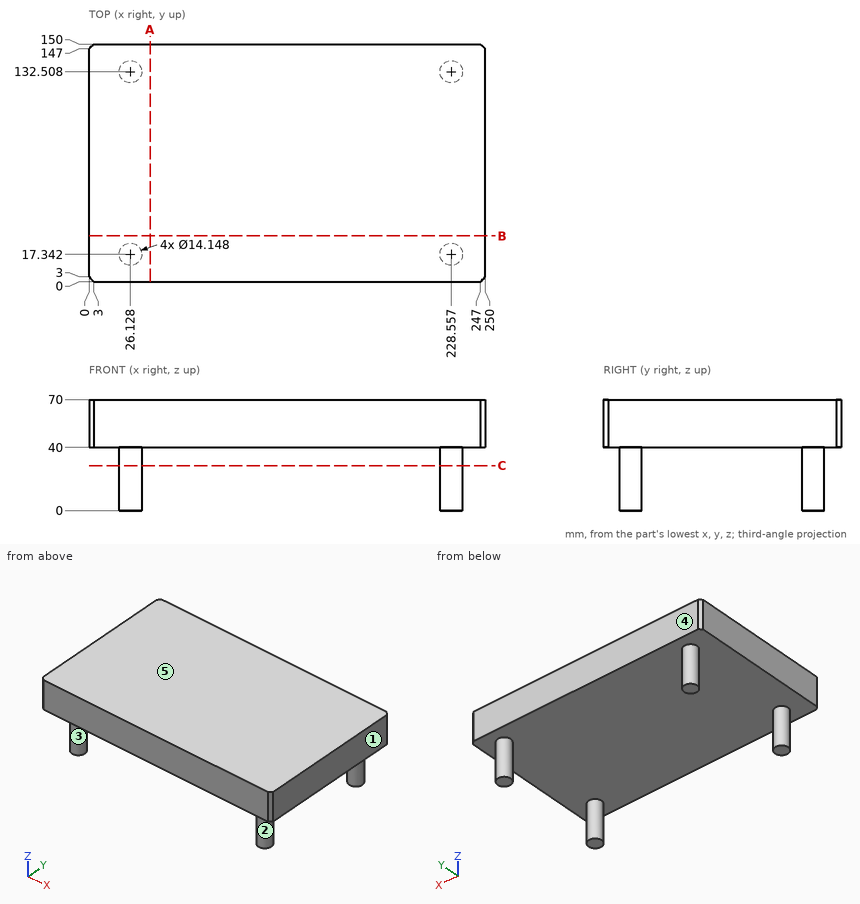
Can you work these out from the drawing? Everything is in mm from the part's minimum corner. A direction names the side the tool comes from. Coordinates: 2 decimals unless noted, no trailing zeros. Write each loop counter-clockwise with the first axis right and the second up, starting at its lowest first coordinate (ties: lowest second). Pieces come first, ordered by that corner, then holes. Notation, with made-up numbers: (40.25, 75) -> (60.25, 75) arc R11 ccw to (60.25, 89) -> close; hole circle Ø1 at (32.5, 79.25). An arc over 180 degrees is marked (long way). Return JSON: item names as keys, results as strings.
(1) Imagine slicing it at C-C, the plane z = 28.5. Please give me the cut outline in (x, y), then the cut area to 3 significant figures.
Numbers:
{"outline": "circle Ø14.15 at (26.13, 17.34); circle Ø14.15 at (26.13, 132.51); circle Ø14.15 at (228.56, 17.34); circle Ø14.15 at (228.56, 132.51)", "area": "629 mm2"}
(2) Imagine slicing it at A-A, the plane x = 38.5. Please give me the cut outline in (y, z), then the cut area to 3 significant figures.
Numbers:
{"outline": "(0, 40) -> (150, 40) -> (150, 70) -> (0, 70) -> close", "area": "4,500 mm2"}
(3) Which directions (+Z, -Z, +X, -X, +Y, -Y) give clear straight access to the entire face, cutting with the end or side of a thin tool? Please do the marked faces 1 and 2.
Numbers:
{"face 1": "+Z, -Z, +X, +Y, -Y", "face 2": "-Z"}
(4) We'd pull the mould along Y, two halves only. Please class the marked faces 3, 4 and 5: +Y half, -Y half, draft (parallel to the pull), parting line (faces both ways), or undercut.
Numbers:
{"face 3": "undercut", "face 4": "+Y half", "face 5": "draft"}
(5) I'm going to push a flat-ended pin straight in: pin 1 (2 mm diameter, centred on x = 109, y = 74, fed in from -Z). Where does the tip first touch, or does it pass through?
Numbers:
{"pin 1": "stops at z = 40"}
(6) Imagine slicing it at B-B, the plane y = 29. Please give me the cut outline in (x, z), then the cut area to 3 significant figures.
Numbers:
{"outline": "(0, 40) -> (250, 40) -> (250, 70) -> (0, 70) -> close", "area": "7,500 mm2"}
(7) I need wall thicknesses on L1, parallel to Z at x = 210, y = 50.5; L2, parallel to X at y = 16.5, z = 14.5; L3, parallel to Y at x = 25, z = 18 (1 decimal). Which ranges of each line are inside material? Lowest first, please.
Numbers:
{"L1": "z = 40 to 70", "L2": "x = 19.1 to 33.15, 221.53 to 235.58", "L3": "y = 10.4 to 24.3, 125.5 to 139.5"}
